```python
from build123d import *

# Parameters (mm, degrees)
SKETCH1_W           = 570
SKETCH1_H           = 620
SKETCH1_W_2         = 25.1
SKETCH1_H_2         = 5.85
SKETCH1_W_3         = 5.85
SKETCH1_H_3         = 25.1
BOSS_EXTRUDE1_DEPTH = 5.8


with BuildPart() as part:
    # Sketch1 → Boss-Extrude1 (new body)
    with BuildSketch(Plane(origin=(0, 0, 0), x_dir=(1, 0, 0), z_dir=(0, 1, 0))):
        Rectangle(SKETCH1_W, SKETCH1_H)
        with Locations((-199.95, 303.075)):
            Rectangle(SKETCH1_W_2, SKETCH1_H_2, mode=Mode.SUBTRACT)
        with Locations((-249.95, 303.075)):
            Rectangle(SKETCH1_W_2, SKETCH1_H_2, mode=Mode.SUBTRACT)
        with Locations((-149.95, 303.075)):
            Rectangle(SKETCH1_W_2, SKETCH1_H_2, mode=Mode.SUBTRACT)
        with Locations((-99.95, 303.075)):
            Rectangle(SKETCH1_W_2, SKETCH1_H_2, mode=Mode.SUBTRACT)
        with Locations((-49.95, 303.075)):
            Rectangle(SKETCH1_W_2, SKETCH1_H_2, mode=Mode.SUBTRACT)
        with Locations((0.05, 303.075)):
            Rectangle(SKETCH1_W_2, SKETCH1_H_2, mode=Mode.SUBTRACT)
        with Locations((50.05, 303.075)):
            Rectangle(SKETCH1_W_2, SKETCH1_H_2, mode=Mode.SUBTRACT)
        with Locations((100.05, 303.075)):
            Rectangle(SKETCH1_W_2, SKETCH1_H_2, mode=Mode.SUBTRACT)
        with Locations((150.05, 303.075)):
            Rectangle(SKETCH1_W_2, SKETCH1_H_2, mode=Mode.SUBTRACT)
        with Locations((200.05, 303.075)):
            Rectangle(SKETCH1_W_2, SKETCH1_H_2, mode=Mode.SUBTRACT)
        with Locations((250.05, 303.075)):
            Rectangle(SKETCH1_W_2, SKETCH1_H_2, mode=Mode.SUBTRACT)
        with Locations((250.05, -303.075)):
            Rectangle(SKETCH1_W_2, SKETCH1_H_2, mode=Mode.SUBTRACT)
        with Locations((200.05, -303.075)):
            Rectangle(SKETCH1_W_2, SKETCH1_H_2, mode=Mode.SUBTRACT)
        with Locations((150.05, -303.075)):
            Rectangle(SKETCH1_W_2, SKETCH1_H_2, mode=Mode.SUBTRACT)
        with Locations((100.05, -303.075)):
            Rectangle(SKETCH1_W_2, SKETCH1_H_2, mode=Mode.SUBTRACT)
        with Locations((50.05, -303.075)):
            Rectangle(SKETCH1_W_2, SKETCH1_H_2, mode=Mode.SUBTRACT)
        with Locations((0.05, -303.075)):
            Rectangle(SKETCH1_W_2, SKETCH1_H_2, mode=Mode.SUBTRACT)
        with Locations((-49.95, -303.075)):
            Rectangle(SKETCH1_W_2, SKETCH1_H_2, mode=Mode.SUBTRACT)
        with Locations((-99.95, -303.075)):
            Rectangle(SKETCH1_W_2, SKETCH1_H_2, mode=Mode.SUBTRACT)
        with Locations((-149.95, -303.075)):
            Rectangle(SKETCH1_W_2, SKETCH1_H_2, mode=Mode.SUBTRACT)
        with Locations((-199.95, -303.075)):
            Rectangle(SKETCH1_W_2, SKETCH1_H_2, mode=Mode.SUBTRACT)
        with Locations((-249.95, -303.075)):
            Rectangle(SKETCH1_W_2, SKETCH1_H_2, mode=Mode.SUBTRACT)
        with Locations((-278.075, 224.95)):
            Rectangle(SKETCH1_W_3, SKETCH1_H_3, mode=Mode.SUBTRACT)
        with Locations((-278.075, 274.95)):
            Rectangle(SKETCH1_W_3, SKETCH1_H_3, mode=Mode.SUBTRACT)
        with Locations((-278.075, 174.95)):
            Rectangle(SKETCH1_W_3, SKETCH1_H_3, mode=Mode.SUBTRACT)
        with Locations((-278.075, 124.95)):
            Rectangle(SKETCH1_W_3, SKETCH1_H_3, mode=Mode.SUBTRACT)
        with Locations((-278.075, 74.95)):
            Rectangle(SKETCH1_W_3, SKETCH1_H_3, mode=Mode.SUBTRACT)
        with Locations((-278.075, 24.95)):
            Rectangle(SKETCH1_W_3, SKETCH1_H_3, mode=Mode.SUBTRACT)
        with Locations((-278.075, -25.05)):
            Rectangle(SKETCH1_W_3, SKETCH1_H_3, mode=Mode.SUBTRACT)
        with Locations((-278.075, -75.05)):
            Rectangle(SKETCH1_W_3, SKETCH1_H_3, mode=Mode.SUBTRACT)
        with Locations((-278.075, -125.05)):
            Rectangle(SKETCH1_W_3, SKETCH1_H_3, mode=Mode.SUBTRACT)
        with Locations((-278.075, -175.05)):
            Rectangle(SKETCH1_W_3, SKETCH1_H_3, mode=Mode.SUBTRACT)
        with Locations((-278.075, -225.05)):
            Rectangle(SKETCH1_W_3, SKETCH1_H_3, mode=Mode.SUBTRACT)
        with Locations((-278.075, -275.05)):
            Rectangle(SKETCH1_W_3, SKETCH1_H_3, mode=Mode.SUBTRACT)
        with Locations((278.075, -274.95)):
            Rectangle(SKETCH1_W_3, SKETCH1_H_3, mode=Mode.SUBTRACT)
        with Locations((278.075, -224.95)):
            Rectangle(SKETCH1_W_3, SKETCH1_H_3, mode=Mode.SUBTRACT)
        with Locations((278.075, -174.95)):
            Rectangle(SKETCH1_W_3, SKETCH1_H_3, mode=Mode.SUBTRACT)
        with Locations((278.075, -124.95)):
            Rectangle(SKETCH1_W_3, SKETCH1_H_3, mode=Mode.SUBTRACT)
        with Locations((278.075, -74.95)):
            Rectangle(SKETCH1_W_3, SKETCH1_H_3, mode=Mode.SUBTRACT)
        with Locations((278.075, -24.95)):
            Rectangle(SKETCH1_W_3, SKETCH1_H_3, mode=Mode.SUBTRACT)
        with Locations((278.075, 25.05)):
            Rectangle(SKETCH1_W_3, SKETCH1_H_3, mode=Mode.SUBTRACT)
        with Locations((278.075, 75.05)):
            Rectangle(SKETCH1_W_3, SKETCH1_H_3, mode=Mode.SUBTRACT)
        with Locations((278.075, 125.05)):
            Rectangle(SKETCH1_W_3, SKETCH1_H_3, mode=Mode.SUBTRACT)
        with Locations((278.075, 175.05)):
            Rectangle(SKETCH1_W_3, SKETCH1_H_3, mode=Mode.SUBTRACT)
        with Locations((278.075, 225.05)):
            Rectangle(SKETCH1_W_3, SKETCH1_H_3, mode=Mode.SUBTRACT)
        with Locations((278.075, 275.05)):
            Rectangle(SKETCH1_W_3, SKETCH1_H_3, mode=Mode.SUBTRACT)
    extrude(amount=BOSS_EXTRUDE1_DEPTH)


solid = part.part
```
Design review of the part built by this model. Coordinates are the model's own, in mm. Round coordinates to 2 decimals unless told otherwise and drop trailing zeros. Order: outer loops, then holes, each group sorted by start corner. A loop starts at its lowest first (then second) coordinate and runs counter-clockwise, first axis right, second up. Notation, with made-up numbers: M -9.5,18.5 L 40.5,18.5 A19 ccw 40.5,43.5 Z; hole C 61.25,-38 d8. An arc over 180 degrees is marked long. Put each result on its own line as item: value.
Q1. To check wall thickness, follow line 1 (Z direction, x = 5.5, y = 1.5); line 2 (X direction, y = 2.75, z = 282). State the ranges of each line that lie inside material, in increasing order.
Reported:
line 1: -310 to -306, -300.15 to 300.15, 306 to 310
line 2: -285 to -281, -275.15 to 275.15, 281 to 285
Q2. Consider section B-B (x = -5). State the section outline as (y, z) points, and give its area (3 significant figures).
Reported:
outline: M 0,-310 L 5.8,-310 L 5.8,-306 L 0,-306 Z; M 0,-300.15 L 5.8,-300.15 L 5.8,300.15 L 0,300.15 Z; M 0,306 L 5.8,306 L 5.8,310 L 0,310 Z
area: 3,530 mm²
Q3. Consider section A-A (z = -23). State the section outline as (x, y) points, and give its area (3 significant figures).
Reported:
outline: M -285,0 L -281,0 L -281,5.8 L -285,5.8 Z; M -275.15,0 L 275.15,0 L 275.15,5.8 L -275.15,5.8 Z; M 281,0 L 285,0 L 285,5.8 L 281,5.8 Z
area: 3,240 mm²
Q4. Consider section C-C (y = 3.7). State how many separate pieces and enclosed holes the cut face has, and give its area (3 significant figures).
Reported:
separate pieces: 1
enclosed holes: 46
area: 347,000 mm²
